The model under review builds one solid part; all positions refer to its coordinate system, in mm. Face numbers are marked on the shaded views. A direction names the side the tool comes from. Give positions to 0.01 mm unless a question says otherwise; leave off trailing zeros. Loops run counter-clockwise (first coordinate to the right, second up) from the corner with the lowest first, then second, coordinate; pieces in that order, holes last. Notation, with made-up numbers: M 47,30.5 L 80,30.5 A22 cw 80,69.5 Z; hole C 5,82 d11. An arc over 180 degrees is marked long. One line per item, written item: value. Start each with the question number.
Q1. Mouldability with a two-part tool opening along Y and no side actions: class the marked faces 1, 2 and 3 as released by +Y, released by -Y, zero draft, split by the parting line, or undercut.
Q2. To check wall thickness, follow line 1 along Y through (x, z) = (2.6, -4); line 2 along X through (y, z) = (18.5, -19); line 3 along Y through (x, z) = (1.75, -19). State the ranges of each line that lie inside material, in increasing order. Write a range as from..to.
Q3. We need section A-A on y = 19. Write out the cut boundary in (x, z).
Q4. We need section B-B on z = -10.5. Write out the cut boundary in (x, y), plus the area to 3 significant figures.
Q5. We need section C-C on z = -16.75. Write out the cut boundary in (x, y).
Q6. We need section D-D on y = 28. Write out the cut boundary in (x, z), plus the area to 3 significant figures.
Q7. For pin 1 (1 mm diameter, centred on x = 4.5, y = 31, fed in from +Z); pin 2 (4 mm diameter, centred on y = 45.5, z = -9, fed in from -X); pin 3 (3 mm diameter, centred on x = 2, z = -1.5, fed in from +Y), all flat-tipped, find the tip position at first contact; note any pin that passes through.
Q8. For the marked faces 4, 5, 6 and 7, list the 3-axis set-ups (+Z, -Z, +X, -X, +Y, -Y) from which the entire face can be reached by the end or side of a thin tool; tool diameter is ignored.
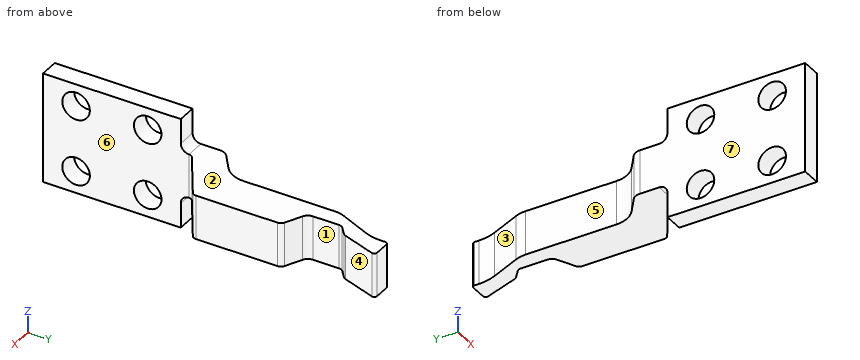
```python
from build123d import *

# Parameters (mm, degrees)
SKETCH1_W                = 20
SKETCH1_H                = 25
BOSS_EXTRUDE2_DEPTH      = 3.5
BOSS_EXTRUDE3_DEPTH      = 9.5
BOSS_EXTRUDE3_DEPTH_BACK = 3.5
SKETCH2_W                = 8
SKETCH2_H                = 41
SKETCH3_R                = 2.5
CUT_EXTRUDE1_DEPTH       = 9.5
CUT_EXTRUDE2_DEPTH       = 9.5
FILLET1_R                = 1.5
FILLET2_R                = 1.5
FILLET3_R                = 2
FILLET4_R                = 5
FILLET5_R                = 5
FILLET6_R                = 8
FILLET7_R                = 0.5
FILLET8_R                = 1
FILLET9_R                = 1
FILLET10_R               = 1
FILLET11_R               = 1.5
FILLET12_R               = 1
FILLET13_R               = 1
FILLET14_R               = 0.5


with BuildPart() as part:
    # Sketch1 → Boss-Extrude2 (new body)
    with BuildSketch(Plane(origin=(0, 0, 0), x_dir=(0, 0, -1), z_dir=(1, 0, 0))):
        with Locations((10, 12.5)):
            Rectangle(SKETCH1_W, SKETCH1_H)
    extrude(amount=BOSS_EXTRUDE2_DEPTH)

    # Sketch2 → Boss-Extrude3 (add, two sides: drawn at the far end of the back side and taken through both)
    with BuildSketch(Plane(origin=(3.5, 0, 0), x_dir=(0, 0, -1), z_dir=(1, 0, 0)).offset(-BOSS_EXTRUDE3_DEPTH_BACK)):
        with Locations((10, 45.5)):
            Rectangle(SKETCH2_W, SKETCH2_H)
    extrude(amount=BOSS_EXTRUDE3_DEPTH + BOSS_EXTRUDE3_DEPTH_BACK)

    # Sketch3 → Cut-Extrude1 (cut)
    with BuildSketch(Plane.ZY):
        with Locations((-16, 19)):
            Circle(SKETCH3_R)
        with Locations((-16, 6)):
            Circle(SKETCH3_R)
        with Locations((-4, 6)):
            Circle(SKETCH3_R)
        with Locations((-4, 19)):
            Circle(SKETCH3_R)
    extrude(amount=-CUT_EXTRUDE1_DEPTH, mode=Mode.SUBTRACT)

    # Sketch4 → Cut-Extrude2 (cut)
    with BuildSketch(Plane.XY.offset(-6)):
        Polygon((0, 66), (0, 31), (5.600462456, 35.199383322), (5.600462456, 55.199383322), (9, 63), (9, 66), align=None)
        Polygon((3.5, 27), (3.5, 25), (13, 25), (13, 33), align=None)
        Polygon((13, 49), (13, 66), (10.600462456, 59.00909695), (8.600462456, 57.318186777), (8.600462456, 51.153091521), align=None)
    extrude(amount=-CUT_EXTRUDE2_DEPTH, mode=Mode.SUBTRACT)

    # Fillet1
    fillet1_edges = [part.edges().sort_by_distance(p)[0] for p in [
        (1.75, 25, -6),
    ]]
    fillet(fillet1_edges, radius=FILLET1_R)

    # Fillet2
    fillet2_edges = [part.edges().sort_by_distance(p)[0] for p in [
        (1.75, 25, -14),
    ]]
    fillet(fillet2_edges, radius=FILLET2_R)

    # Fillet3
    fillet3_edges = [part.edges().sort_by_distance(p)[0] for p in [
        (0, 31, -10),
    ]]
    fillet(fillet3_edges, radius=FILLET3_R)

    # Fillet4
    fillet4_edges = [part.edges().sort_by_distance(p)[0] for p in [
        (5.600462456, 35.199383322, -10),
    ]]
    fillet(fillet4_edges, radius=FILLET4_R)

    # Fillet5
    fillet5_edges = [part.edges().sort_by_distance(p)[0] for p in [
        (5.600462456, 55.199383322, -10),
    ]]
    fillet(fillet5_edges, radius=FILLET5_R)

    # Fillet6
    fillet6_edges = [part.edges().sort_by_distance(p)[0] for p in [
        (9, 63, -10),
    ]]
    fillet(fillet6_edges, radius=FILLET6_R)

    # Fillet7
    fillet7_edges = [part.edges().sort_by_distance(p)[0] for p in [
        (9, 66, -10),
    ]]
    fillet(fillet7_edges, radius=FILLET7_R)

    # Fillet8
    fillet8_edges = [part.edges().sort_by_distance(p)[0] for p in [
        (3.5, 27, -10),
    ]]
    fillet(fillet8_edges, radius=FILLET8_R)

    # Fillet9
    fillet9_edges = [part.edges().sort_by_distance(p)[0] for p in [
        (13, 33, -10),
    ]]
    fillet(fillet9_edges, radius=FILLET9_R)

    # Fillet10
    fillet10_edges = [part.edges().sort_by_distance(p)[0] for p in [
        (13, 49, -10),
    ]]
    fillet(fillet10_edges, radius=FILLET10_R)

    # Fillet11
    fillet11_edges = [part.edges().sort_by_distance(p)[0] for p in [
        (8.600462456, 51.153091521, -10),
    ]]
    fillet(fillet11_edges, radius=FILLET11_R)

    # Fillet12
    fillet12_edges = [part.edges().sort_by_distance(p)[0] for p in [
        (8.600462456, 57.318186777, -10),
    ]]
    fillet(fillet12_edges, radius=FILLET12_R)

    # Fillet13
    fillet13_edges = [part.edges().sort_by_distance(p)[0] for p in [
        (10.600462456, 59.00909695, -10),
    ]]
    fillet(fillet13_edges, radius=FILLET13_R)

    # Fillet14
    fillet14_edges = [part.edges().sort_by_distance(p)[0] for p in [
        (13, 66, -10),
    ]]
    fillet(fillet14_edges, radius=FILLET14_R)


solid = part.part
```
Solved:
1. face 1: undercut
1. face 2: zero draft
1. face 3: released by +Y
2. line 1: 0..3.5, 8.5..16.5, 21.5..25
2. line 2: 0..3.5
2. line 3: 0..25
3. outline: M 0,-20 L 3.5,-20 L 3.5,-18.5 L 0,-18.5 Z; M 0,-13.5 L 3.5,-13.5 L 3.5,-6.5 L 0,-6.5 Z; M 0,-1.5 L 3.5,-1.5 L 3.5,0 L 0,0 Z
4. outline: M 0,0 L 3.5,0 L 3.5,26.45 A1 cw 3.97,27.29 L 12.53,32.71 A1 ccw 13,33.55 L 13,48.38 A1 ccw 12.44,49.27 L 9.44,50.74 A1.5 cw 8.6,52.09 L 8.6,56.85 A1 cw 8.95,57.62 L 10.39,58.83 A1 ccw 10.69,59.27 L 12.77,65.34 A0.5 ccw 12.3,66 L 9.5,66 A0.5 ccw 9,65.5 L 9,64.67 A8 cw 8.33,61.47 L 6.02,56.15 A5 ccw 5.6,54.16 L 5.6,37.7 A5 cw 3.6,33.7 L 0.8,31.6 A2 ccw 0,30 Z
4. area: 320 mm2
5. outline: M 0,0 L 3.5,0 L 3.5,3.62 L 0,3.62 Z; M 0,8.38 L 3.5,8.38 L 3.5,16.62 L 0,16.62 Z; M 0,21.38 L 3.5,21.38 L 3.5,25 L 0,25 Z
6. outline: M 0,-14 L 5.08,-14 L 5.08,-6 L 0,-6 Z
6. area: 40.7 mm2
7. pin 1: z = -6
7. pin 2: x = 5.6
7. pin 3: y = 25
8. face 4: +Z, -Z, +X
8. face 5: +Z, -Z, -X, +Y
8. face 6: +Z, -Z, +X, -Y
8. face 7: +Z, -Z, -X, +Y, -Y
